from build123d import *

# Parameters (mm, degrees)
F0_R     = 2.5
F1_DEPTH = 3
F2_DEPTH = 5
F3_DEPTH = 7
F4_DEPTH = 2
F5_R     = 0.75
F5_R_2   = 0.7
F6_DEPTH = 25
F7_R     = 1


with BuildPart() as f1:
    # F0 (on Top) → F1 (new body)
    with BuildSketch(Plane.XY):
        with BuildLine():
            Line((-36.539011, -10), (0, -10))
            Line((0, -10), (36.539011, -10))
            ThreePointArc((36.539011, -10), (47.491782, 0.473014), (35.706888, 10))
            Line((35.706888, 10), (0, 10))
            Line((0, 10), (-35.706888, 10))
            ThreePointArc((-35.706888, 10), (-47.491782, 0.473014), (-36.539011, -10))
        make_face()
        with Locations((-43.000363, 0)):
            Circle(F0_R, mode=Mode.SUBTRACT)
        with BuildLine():
            Line((33.603549, -6), (0, -6))
            Line((0, -6), (-33.603549, -6))
            ThreePointArc((-33.603549, -6), (-38.405942, -0.153092), (-34.002674, 6))
            Line((-34.002674, 6), (0, 6))
            Line((0, 6), (34.002674, 6))
            ThreePointArc((34.002674, 6), (38.405942, -0.153092), (33.603549, -6))
        make_face(mode=Mode.SUBTRACT)
        with Locations((43.000363, 0)):
            Circle(F0_R, mode=Mode.SUBTRACT)
    extrude(amount=F1_DEPTH)

    # F0 (on Top) → F2 (join)
    with BuildSketch(Plane.XY):
        with BuildLine():
            Line((-33.603549, -6), (0, -6))
            Line((0, -6), (33.603549, -6))
            ThreePointArc((33.603549, -6), (38.405942, -0.153092), (34.002674, 6))
            Line((34.002674, 6), (0, 6))
            Line((0, 6), (-34.002674, 6))
            ThreePointArc((-34.002674, 6), (-38.405942, -0.153092), (-33.603549, -6))
        make_face()
        with BuildLine():
            Line((-33.847273, 5), (0, 5))
            Line((0, 5), (33.847273, 5))
            ThreePointArc((33.847273, 5), (37.405931, -0.136053), (33.483545, -5))
            Line((33.483545, -5), (0, -5))
            Line((0, -5), (-33.483545, -5))
            ThreePointArc((-33.483545, -5), (-37.405931, -0.136053), (-33.847273, 5))
        make_face(mode=Mode.SUBTRACT)
    extrude(amount=F2_DEPTH)

    # F0 (on Top) → F3 (join)
    with BuildSketch(Plane.XY):
        with BuildLine():
            Line((33.847273, 5), (0, 5))
            Line((0, 5), (-33.847273, 5))
            ThreePointArc((-33.847273, 5), (-37.405931, -0.136053), (-33.483545, -5))
            Line((-33.483545, -5), (0, -5))
            Line((0, -5), (33.483545, -5))
            ThreePointArc((33.483545, -5), (37.405931, -0.136053), (33.847273, 5))
        make_face()
        with BuildLine():
            Line((33.351164, -4), (0, -4))
            Line((0, -4), (-33.351164, -4))
            ThreePointArc((-33.351164, -4), (-36.405914, -0.117327), (-33.675664, 4))
            Line((-33.675664, 4), (0, 4))
            Line((0, 4), (33.675664, 4))
            ThreePointArc((33.675664, 4), (36.405914, -0.117327), (33.351164, -4))
        make_face(mode=Mode.SUBTRACT)
    extrude(amount=F3_DEPTH)

    # F0 (on Top) → F4 (join)
    with BuildSketch(Plane.XY):
        with BuildLine():
            Line((-33.351164, -4), (0, -4))
            Line((0, -4), (33.351164, -4))
            ThreePointArc((33.351164, -4), (36.405914, -0.117327), (33.675664, 4))
            Line((33.675664, 4), (0, 4))
            Line((0, 4), (-33.675664, 4))
            ThreePointArc((-33.675664, 4), (-36.405914, -0.117327), (-33.351164, -4))
        make_face()
    extrude(amount=F4_DEPTH)

    # F5 (on face) → F6 (cut)
    with BuildSketch(Plane.XY.offset(2)):
        with BuildLine():
            ThreePointArc((0, 0.75), (-0.75, 0), (0, -0.75))
            ThreePointArc((0, -0.75), (0.75, 0), (0, 0.75))
        make_face()
        with BuildLine():
            ThreePointArc((0, 3.25), (-0.75, 2.5), (0, 1.75))
            ThreePointArc((0, 1.75), (0.75, 2.5), (0, 3.25))
        make_face()
        with Locations((2.5, 0)):
            Circle(F5_R)
        with Locations((2.5, 2.5)):
            Circle(F5_R)
        with Locations((5, 0)):
            Circle(F5_R)
        with Locations((5, 2.5)):
            Circle(F5_R)
        with Locations((7.5, 0)):
            Circle(F5_R)
        with Locations((7.5, 2.5)):
            Circle(F5_R)
        with Locations((10, 0)):
            Circle(F5_R)
        with Locations((10, 2.5)):
            Circle(F5_R)
        with Locations((12.5, 0)):
            Circle(F5_R)
        with Locations((12.5, 2.5)):
            Circle(F5_R)
        with Locations((15, 0)):
            Circle(F5_R)
        with Locations((15, 2.5)):
            Circle(F5_R)
        with Locations((17.5, 0)):
            Circle(F5_R)
        with Locations((17.5, 2.5)):
            Circle(F5_R)
        with Locations((20, 0)):
            Circle(F5_R)
        with Locations((20, 2.5)):
            Circle(F5_R)
        with Locations((22.5, 0)):
            Circle(F5_R)
        with Locations((22.5, 2.5)):
            Circle(F5_R)
        with Locations((25, 0)):
            Circle(F5_R)
        with Locations((25, 2.5)):
            Circle(F5_R)
        with Locations((2.5, -2.5)):
            Circle(F5_R)
        with Locations((5, -2.5)):
            Circle(F5_R)
        with Locations((7.5, -2.5)):
            Circle(F5_R)
        with Locations((10, -2.5)):
            Circle(F5_R)
        with Locations((12.5, -2.5)):
            Circle(F5_R)
        with Locations((15, -2.5)):
            Circle(F5_R)
        with Locations((17.5, -2.5)):
            Circle(F5_R)
        with Locations((20, -2.5)):
            Circle(F5_R)
        with Locations((22.5, -2.5)):
            Circle(F5_R)
        with Locations((25, -2.5)):
            Circle(F5_R)
        with Locations((27.5, 0)):
            Circle(F5_R)
        with Locations((27.5, -2.5)):
            Circle(F5_R)
        with Locations((-12.5, 0)):
            Circle(F5_R)
        with Locations((-17.5, 0)):
            Circle(F5_R)
        with Locations((-7.5, 0)):
            Circle(F5_R)
        with Locations((-5, 0)):
            Circle(F5_R)
        with Locations((-15, 0)):
            Circle(F5_R)
        with Locations((-20, 0)):
            Circle(F5_R)
        with Locations((-10, 0)):
            Circle(F5_R)
        with Locations((-12.5, 2.5)):
            Circle(F5_R)
        with Locations((-10, 2.5)):
            Circle(F5_R)
        with Locations((-7.5, 2.5)):
            Circle(F5_R)
        with Locations((-5, 2.5)):
            Circle(F5_R)
        with Locations((-2.5, 0)):
            Circle(F5_R)
        with Locations((-2.5, 2.5)):
            Circle(F5_R)
        with Locations((-17.5, 2.5)):
            Circle(F5_R)
        with Locations((-15, 2.5)):
            Circle(F5_R)
        with Locations((-20, 2.5)):
            Circle(F5_R)
        with Locations((-27.5, 0)):
            Circle(F5_R)
        with Locations((-22.5, 0)):
            Circle(F5_R)
        with Locations((-25, 0)):
            Circle(F5_R)
        with Locations((-27.5, -2.5)):
            Circle(F5_R)
        with Locations((-25, 2.5)):
            Circle(F5_R)
        with Locations((-22.5, 2.5)):
            Circle(F5_R)
        with Locations((-17.5, -2.5)):
            Circle(F5_R)
        with Locations((-27.5, 2.5)):
            Circle(F5_R)
        with Locations((-20, -2.5)):
            Circle(F5_R)
        with Locations((-22.5, -2.5)):
            Circle(F5_R)
        with Locations((-25, -2.5)):
            Circle(F5_R)
        with Locations((-2.5, -2.5)):
            Circle(F5_R)
        with Locations((-5, -2.5)):
            Circle(F5_R)
        with Locations((-7.5, -2.5)):
            Circle(F5_R)
        with Locations((-10, -2.5)):
            Circle(F5_R)
        with Locations((-12.5, -2.5)):
            Circle(F5_R)
        with Locations((-15, -2.5)):
            Circle(F5_R)
        with Locations((0.020794, -2.485011)):
            Circle(F5_R_2)
        with Locations((-29.956931, 0.036661)):
            Circle(F5_R)
        with Locations((29.956931, 0.036661)):
            Circle(F5_R)
        with Locations((30, -2.5)):
            Circle(F5_R)
        with Locations((32.5, 0)):
            Circle(F5_R)
        with Locations((32.5, -2.5)):
            Circle(F5_R)
        with Locations((35, 0)):
            Circle(F5_R)
        with Locations((27.5, 2.5)):
            Circle(F5_R)
        with Locations((30, 2.5)):
            Circle(F5_R)
        with Locations((32.5, 2.5)):
            Circle(F5_R)
        with Locations((-30, 2.5)):
            Circle(F5_R)
        with Locations((-32.5, 0)):
            Circle(F5_R)
        with Locations((-30, -2.5)):
            Circle(F5_R)
        with Locations((-32.5, -2.5)):
            Circle(F5_R)
        with Locations((-32.5, 2.5)):
            Circle(F5_R)
        with Locations((-35, 0)):
            Circle(F5_R)
    extrude(amount=-F6_DEPTH, mode=Mode.SUBTRACT)

    # F7
    f7_edges = [f1.edges().sort_by_distance(p)[0] for p in [
        (-45.500363, 0, 3),
        (40.500363, 0, 3),
    ]]
    fillet(f7_edges, radius=F7_R)


solid = f1.part
Check sheet for the modelled part. Datum: model origin and axes. Units: mm. A direction names the side the tool comes from. Give positions to 0.01 mm unless a question says otherwise; leave off trailing zeros. Write each loop counter-clockwise with the first axis right and the second up, starting at its lowest first coordinate (ties: lowest second). Pieces come first, ordered by that corner, then holes. Notation, with made-up numbers: (43, 61) -> (47, 61) arc R28 cw to (47, 98) -> close; hole circle Ø9 at (-37, -14). An arc over 180 degrees is marked (long way). Write item = value, one per line.
Item 1: Sectioned sample at C-C on y = -7.25. Record the boundary of the cut face in (x, z).
Output:
outline = (-44.37, 0) -> (44.37, 0) -> (44.37, 3) -> (-44.37, 3) -> close
Item 2: Sectioned sample at A-A on z = 1. Count the separate pieces of the cut face and the enclosed holes in it, and give its area (3 significant figures).
Output:
separate_pieces = 1
enclosed_holes = 85
area = 1,630 mm^2
Item 3: Release check for a two-part mould opening along X. For faces 1 (the cylindrical face through (-37.41, -0.04, 5.99)), 2 (the cylindrical face through (-20.75, 0.03, 1.01)), 3 (the flat face through (0, -6, 4)) record: +X half, -X half, draft (parallel to the pull), parting line (faces both ways), or undercut.
Output:
face_1 = -X half
face_2 = undercut
face_3 = draft
Item 4: Gauge pin test, flat ends, axial feed: pin 1 (1.4 mm diameter, centred on x = 22.5, y = 2.5, fed in from +Z); pin 2 (4 mm diameter, centred on y = 2.5, z = 3, fed in from -X); pin 3 (2.5 mm diameter, centred on x = 27.5, y = 0, fed in from +Z); pin 4 (4 mm diameter, centred on x = -0.5, z = 2.5, fed in from +Y). Record the tip position at first contact, or that the pin passes through.
Output:
pin_1 = through
pin_2 = -47.49
pin_3 = 2
pin_4 = 10
Item 5: Scan lines: probe 1 along Y at (x, z) = (27.5, 1); probe 2 along Y at (x, z) = (-33, 3.25); probe 3 along Y at (x, z) = (-26, 5.75). Record each from-to range of solid material in increasing order. Write a range as from..to.
Output:
probe_1 = -10..-3.25, -1.75..-0.75, 0.75..1.75, 3.25..10
probe_2 = -6..-4, 4..6
probe_3 = -5..-4, 4..5
Item 6: Sectioned sample at B-B on y = 8.5. Record the boundary of the cut face in (x, z).
Output:
outline = (-42.93, 0) -> (42.93, 0) -> (42.93, 3) -> (-42.93, 3) -> close
Item 7: Tool access check on faces 4 (the cylindrical face through (-13.25, 0.03, 1.01)), 5 (the flat face through (0, 5, 6)), 6 (the flat face through (-1, -1, 2)). Record the directions out of +Z, -Z, +X, -X, +Y, -Y that give a thin tool (end or side, any length) a straight path to the whole face; none if there is none.
Output:
face_4 = +Z, -Z
face_5 = +Z, +X, -X, +Y
face_6 = +Z
